Read the model definition and answer for the solid it produces. Units are mm, in the model's axes. A direction names the side the tool comes from. Coordinates: 2 decimals unless noted, no trailing zeros. Order: outer loops, then holes, each group sorted by start corner. A loop starts at its lowest first (then second) coordinate and runs counter-clockwise, first axis right, second up. Notation, with made-up numbers: M 59.5,-26 L 70.5,-26 A25 cw 70.5,13 Z; hole C -30,86 d8. An arc over 180 degrees is marked long. Use a Markdown table: item, result. Add a question column.
1) The mould has two halves that part along X. Classify faces 4 (the face through (-5, 0, 6)), 5 (the face through (15.517, 4.514, 3.5)), 6 (the face through (-21.76, -2.86, 4.37)), 7 (the face through (-18.2, -4, 1)): released by +X, released by -X, zero draft, split by the parting line, or undercut.
2) Find section C-C on x = -29.5. Write down the section's boundary in (y, z).
3) Find the intervals of material crossed by probe 1 along X at (y, z) = (1.5, 5.5); probe 2 along X at (y, z) = (-2.5, 0.5); probe 3 along Y at (x, z) = (-14, 3.75), in increasing order. Write a range as [from, to].
4) Find section A-A on x = 12. Write down the section's boundary in (y, z), plus the area to 3 significant figures.
5) For faces 1 (the face through (-28.71, -3.06, 2.51)), 2 (the face through (22, -0.5, 3)), 3 (the face through (0, -1, 2)), determine the directions among +Z, -Z, +X, -X, +Y, -Y from which every point of the face is accessible in a straight line to the end or side of a thin tool.
6) Each of these flat-tipped pins is pushed along its axis until it touches: pin 1 Ø3 at (x, z) = (3.5, 2.5) entering from +Y; pin 2 Ø1.5 at (y, z) = (-2.5, 2.5) entering from +X. Where does it stop, or does it pass through?
7) Find section B-B on x = -8. Write down the section's boundary in (y, z).
from build123d import *

# Parameters (mm, degrees)
SKETCH_1_W          = 70.4
SKETCH_1_H          = 11
EXTRUDE_1_DEPTH     = 6
CUT_EXTRUDE_1_DEPTH = 6.5
CUT_EXTRUDE_3_DEPTH = 17
CUT_EXTRUDE_4_DEPTH = 2
CUT_EXTRUDE_5_DEPTH = 12
CUT_EXTRUDE_6_DEPTH = 7
SKETCH_11_R         = 2.5
CUT_EXTRUDE_7_DEPTH = 9.52081528


with BuildPart() as part:
    # Эскиз1 → Бобышка-Вытянуть1 (new body)
    with BuildSketch(Plane.XY):
        Rectangle(SKETCH_1_W, SKETCH_1_H)
    extrude(amount=EXTRUDE_1_DEPTH)

    # Эскиз3 → Вырез-Вытянуть1 (cut)
    with BuildSketch(Plane(origin=(0, 5.5, 0), x_dir=(1, 0, 0), z_dir=(0, 1, 0))):
        with BuildLine():
            Line((13.564659966, 0), (-13.564659966, 0))
            ThreePointArc((-13.564659966, 0), (0, -4), (13.564659966, 0))
        make_face()
    extrude(amount=-CUT_EXTRUDE_1_DEPTH, mode=Mode.SUBTRACT)

    # Эскиз6 → Вырез-Вытянуть3 (cut)
    with BuildSketch(Plane.ZY.offset(35.2)):
        Polygon((4.949747468, -5.5), (0, -0.550252532), (0, -5.5), align=None)
    extrude(amount=-CUT_EXTRUDE_3_DEPTH, mode=Mode.SUBTRACT)

    # Эскиз7 → Вырез-Вытянуть4 (cut)
    with BuildSketch(Plane(origin=(0, 5.5, 0), x_dir=(1, 0, 0), z_dir=(0, 1, 0))):
        with BuildLine():
            Line((-13.564659966, 0), (-20, 0))
            ThreePointArc((-20, 0), (-15.583005244, -3.457513111), (-10.583005244, -6))
            Line((-10.583005244, -6), (10.583005244, -6))
            ThreePointArc((10.583005244, -6), (15.583005244, -3.457513111), (20, 0))
            Line((20, 0), (13.564659966, 0))
            ThreePointArc((13.564659966, 0), (0, -4), (-13.564659966, 0))
        make_face()
    extrude(amount=-CUT_EXTRUDE_4_DEPTH, mode=Mode.SUBTRACT)

    # Эскиз9 → Вырез-Вытянуть5 (cut, through all)
    with BuildSketch(Plane(origin=(0, 5.5, 0), x_dir=(1, 0, 0), z_dir=(0, 1, 0))):
        Polygon((26.8, 134.579292019), (26.8, 0), (26.8, -6), (26.8, -140.579292019), (295.958584038, -140.579292019), (295.958584038, 134.579292019), align=None)
    extrude(amount=-CUT_EXTRUDE_5_DEPTH, mode=Mode.SUBTRACT)

    # Эскиз10 → Вырез-Вытянуть6 (cut, through all)
    with BuildSketch(Plane.XY.offset(6)):
        Polygon((16.8, -140.079292019), (16.8, -5.5), (16.8, -0.5), (26.8, -0.5), (161.379292019, -0.5), (348.325311663, -194.142787371), (203.746019644, -333.72207939), align=None)
    extrude(amount=-CUT_EXTRUDE_6_DEPTH, mode=Mode.SUBTRACT)

    # Эскиз11 → Вырез-Вытянуть7 (cut, through all)
    with BuildSketch(Plane(origin=(0, -0.275126266, -0.275126266), x_dir=(1, 0, 0), z_dir=(0, -0.707106781, -0.707106781))):
        with Locations((-26.2, 2.610912703)):
            Circle(SKETCH_11_R)
        with Locations((-30.7, 7.610912703)):
            Circle(SKETCH_11_R)
        with Locations((-21.7, 7.610912703)):
            Circle(SKETCH_11_R)
    extrude(amount=-CUT_EXTRUDE_7_DEPTH, mode=Mode.SUBTRACT)


solid = part.part
Check result:
| question | item | result |
|---|---|---|
| 1 | face 4 | zero draft |
| 1 | face 5 | undercut |
| 1 | face 6 | undercut |
| 1 | face 7 | released by -X |
| 2 | outline | M -4.11,3.56 L -0.55,0 L 5.5,0 L 5.5,6 L -1.66,6 Z |
| 3 | probe 1 | x = [-35.2, -28.69], [-23.71, 26.8] |
| 3 | probe 2 | x = [-18.2, 16.8] |
| 3 | probe 3 | y = [-5.5, 3.5] |
| 4 | outline | M -5.5,0 L -1,0 L -1,0.93 L 3.5,0.93 L 3.5,5.4 L 5.5,5.4 L 5.5,6 L -5.5,6 Z |
| 4 | area | 51.0 mm2 |
| 5 | face 1 | -Z, -X, -Y |
| 5 | face 2 | +Z, -Z, +X, -Y |
| 5 | face 3 | -Z, +Y |
| 6 | pin 1 | stops at y = 3.5 |
| 6 | pin 2 | stops at x = 16.8 |
| 7 | outline | M -5.5,0 L -1,0 L -1,2.69 L 3.5,2.69 L 3.5,6 L -5.5,6 Z |
